Source: CAD feature listing. Evaluate the final solid. Frame: model axes, mm. A direction names the side the tool comes from. Coordinates: 2 decimals unless noted, no trailing zeros. Loops run counter-clockwise (first coordinate to the right, second up) from the corner with the lowest first, then second, coordinate; pieces in that order, holes last.
Item 1: Section query D-D, the plane y = -231.5. Return the cut outline in (x, z).
Item 2: Section query C-C, the plane x = 213. Return the cut outline in (y, z), then the cut area to 3 significant figures.
Item 3: Pull-direction query (X, two-part tool) for faces 6 (the flat face through (217, -156.1, 1)), 7 (the flat face through (211.157, -155, 1)), 8 (the flat face through (186.757, -259, 1)); classes: +X half, -X half, draft (parallel to the pull), parting line (faces both ways), or undercut.
Item 4: Section query A-A, the plane x = 182.5. Return the cut outline in (y, z), then the cut area to 3 significant figures.
Item 5: Line query: probe 1 along X at (y, z) = (-216.5, 2.6); probe 2 along Y at (x, z) = (188, 0.35); probe 3 along X at (y, z) = (-164.5, 1.25). Output: solid intervals per line, ascending.
Item 6: Reachability of faces 1 (the flat face through (198.957, -259, 1)), 2 (the flat face through (223.357, -255, 1)), 3 (the flat face through (225, -247.71, 1)), 4 (the flat face through (165.357, -221, 1)), 5 (the flat face through (170, -257.71, 1)) from +Z, -Z, +X, -X, +Y, -Y: full face, straight path, thin tool, end or side. Return the list, or none.
Item 7: Section query B-B, the plane y = -179.5. Return the cut outline in (x, z).
Item 8: Pin query (flat end, axial travel): pin 1 Ø1.5 at (x, z) = (168.5, 2) entering from +Y; pin 2 Ø0.9 at (x, z) = (215, 2) entering from -Y; pin 3 Ø0.9 at (y, z) = (-247, 1) entering from -X. Return the tip coordinate at first contact, or that it passes through.
```python
from build123d import *

# Parameters (mm, degrees)
CROQUIS1_R              = 5
SALIENTE_EXTRUIR1_DEPTH = 3


with BuildPart() as part:
    # Croquis1 → Saliente-Extruir1 (new body)
    with BuildSketch(Plane.XY):
        Polygon((174.557067775, -156.100114598), (165.357067775, -156.100114598), (165.357067775, -170.615828883), (162.357067775, -170.615828883), (162.357067775, -185.131543169), (165.357067775, -185.131543169), (165.357067775, -199.647257455), (162.357067775, -199.647257455), (162.357067775, -214.162971741), (165.357067775, -214.162971741), (165.357067775, -228.678686026), (162.357067775, -228.678686026), (162.357067775, -243.194400312), (165.357067775, -243.194400312), (165.357067775, -257.710114598), (174.557067775, -257.710114598), (174.557067775, -260.710114598), (186.757067775, -260.710114598), (186.757067775, -257.710114598), (198.957067775, -257.710114598), (198.957067775, -260.710114598), (211.157067775, -260.710114598), (211.157067775, -257.710114598), (223.357067775, -257.710114598), (223.357067775, -252.710114598), (226.776809623, -252.710114598), (226.776809623, -247.710114598), (223.357067775, -247.710114598), (223.357067775, -170.615828883), (223.357067775, -166.100114598), (226.776809623, -166.100114598), (226.776809623, -161.100114598), (223.357067775, -161.100114598), (223.357067775, -156.100114598), (211.157067775, -156.100114598), (211.157067775, -153.100114598), (198.957067775, -153.100114598), (198.957067775, -156.100114598), (186.757067775, -156.100114598), (186.757067775, -153.100114598), (174.557067775, -153.100114598), align=None)
        with Locations((179.628110515, -177.498140377)):
            Circle(CROQUIS1_R, mode=Mode.SUBTRACT)
    extrude(amount=SALIENTE_EXTRUIR1_DEPTH)


solid = part.part
```
Verdict:
1. outline: (162.36, 0) - (223.36, 0) - (223.36, 3) - (162.36, 3) - close
2. outline: (-257.71, 0) - (-156.1, 0) - (-156.1, 3) - (-257.71, 3) - close
2. area: 305 mm2
3. face 6: draft
3. face 7: +X half
3. face 8: undercut
4. outline: (-260.71, 0) - (-181.59, 0) - (-181.59, 3) - (-260.71, 3) - close; (-173.41, 0) - (-153.1, 0) - (-153.1, 3) - (-173.41, 3) - close
4. area: 298 mm2
5. probe 1: x = 165.36 to 223.36
5. probe 2: y = -257.71 to -156.1
5. probe 3: x = 165.36 to 226.78
6. face 1: +Z, -Z, -Y
6. face 2: +Z, -Z, +X, -Y
6. face 3: +Z, -Z, +X
6. face 4: +Z, -Z, -X
6. face 5: +Z, -Z, -X, -Y
7. outline: (162.36, 0) - (175.05, 0) - (175.05, 3) - (162.36, 3) - close; (184.21, 0) - (223.36, 0) - (223.36, 3) - (184.21, 3) - close
8. pin 1: stops at y = -156.1
8. pin 2: stops at y = -257.71
8. pin 3: stops at x = 165.36
